from build123d import *

# Parameters (mm, degrees)
ESQUISSE3_R                         = 14.8
BOSS_EXTRU_1_DEPTH                  = 2
BOSS_EXTRU_2_REACH                  = 31.138
R_P_TITION_CIRCULAIRE1_COUNT        = 3
ENL_V_MAT_EXTRU_1_DEPTH             = 30.137604569
ENL_V_MAT_EXTRU_1_DEPTH_BACK        = 30.137604569
ESQUISSE5_R                         = 1.625
PER_AGEAVANC_1_START                = -3.4
PER_AGEAVANC_1_OUTLINE_R            = 3
PER_AGEAVANC_1_OUTLINE_R_2          = 1.625
PER_AGEAVANC_1_DEPTH                = 3.4000121
ENL_V_MAT_EXTRU_2_DEPTH             = 1
ENL_V_MAT_EXTRU_2_DRAFT             = -43
R_P_TITION_CIRCULAIRE2_COPY_1_DEPTH = 1
R_P_TITION_CIRCULAIRE2_COPY_1_DRAFT = -43
R_P_TITION_CIRCULAIRE2_COPY_2_DEPTH = 1
R_P_TITION_CIRCULAIRE2_COPY_2_DRAFT = -43
R_P_TITION_CIRCULAIRE2_COPY_3_DEPTH = 1
R_P_TITION_CIRCULAIRE2_COPY_3_DRAFT = -43


with BuildPart() as part:
    # Esquisse2 → Révolution1 (revolve)
    with BuildSketch(Plane(origin=(0, 0, 0), x_dir=(0, 0, -1), z_dir=(1, 0, 0)), mode=Mode.PRIVATE) as r_volution1_sk:
        Polygon((0, 0), (0, 20), (5, 15), (5, 0), align=None)
    revolve(r_volution1_sk.sketch.rotate(Axis((0, 0, 0), (0, 0, -1)), 90), axis=Axis((0, 0, 0), (0, 0, -1)))

    # Esquisse3 → Boss.-Extru.1 (add)
    with BuildSketch(Plane(origin=(0, 0, -5), x_dir=(-1, 0, 0), z_dir=(0, 0, -1))):
        Circle(ESQUISSE3_R)
    extrude(amount=BOSS_EXTRU_1_DEPTH)

    # Boss.-Extru.2: up to this face of the body (flat: up to its plane)
    boss_extru_2_end = Plane(part.part.faces().sort_by_distance((0, 0, -7))[0])
    # Esquisse4 → Boss.-Extru.2 (add, up to the picked face)
    with BuildSketch(Plane.XY, mode=Mode.PRIVATE) as boss_extru_2_sk1:
        with BuildLine():
            Line((1.5, 19.943670675), (-1.5, 19.943670675))
            Line((-1.5, 19.943670675), (-3.52737474, 14.373504355))
            ThreePointArc((-3.52737474, 14.373504355), (0, 14.8), (3.52737474, 14.373504355))
            Line((3.52737474, 14.373504355), (1.5, 19.943670675))
        make_face()
    boss_extru_2_tool1 = split(extrude(boss_extru_2_sk1.sketch, amount=-BOSS_EXTRU_2_REACH, mode=Mode.PRIVATE), bisect_by=boss_extru_2_end, keep=Keep.BOTH, mode=Mode.PRIVATE)
    boss_extru_2 = boss_extru_2_tool1.solids().sort_by(Axis((0, 16.957577, 0), (0, 0, -1)))[0]
    add(boss_extru_2)

    # Répétition circulaire1: Boss.-Extru.2 ×3 about axis
    r_p_tition_circulaire1_axis = Axis((0, 0, 0), (0, 0, 1))
    for i in range(1, R_P_TITION_CIRCULAIRE1_COUNT):
        add(boss_extru_2.rotate(r_p_tition_circulaire1_axis, i * 360 / R_P_TITION_CIRCULAIRE1_COUNT))

    # Esquisse5 → Enlèv. mat.-Extru.1 (cut, two sides: drawn at the far end of the back side and taken through both)
    with BuildSketch(Plane.XY.offset(-ENL_V_MAT_EXTRU_1_DEPTH_BACK)):
        with Locations((0, 7)):
            Circle(ESQUISSE5_R)
        Circle(ESQUISSE5_R)
        with Locations((7, 0)):
            Circle(ESQUISSE5_R)
        with Locations((0, -7)):
            Circle(ESQUISSE5_R)
        with Locations((-7, 0)):
            Circle(ESQUISSE5_R)
    extrude(amount=ENL_V_MAT_EXTRU_1_DEPTH + ENL_V_MAT_EXTRU_1_DEPTH_BACK, mode=Mode.SUBTRACT)

    # PerçageAvancé1: read off the stored shape, not the designer's step
    # PerçageAvancé1 outline → PerçageAvancé1 (cut)
    # profile 1 of 5: a face of its own
    with BuildSketch(Plane.XY.offset(PER_AGEAVANC_1_START)):
        with Locations((0, -7)):
            Circle(PER_AGEAVANC_1_OUTLINE_R)
        with Locations((0, -7)):
            Circle(PER_AGEAVANC_1_OUTLINE_R_2, mode=Mode.SUBTRACT)
    # profile 2 of 5: a face of its own
    with BuildSketch(Plane.XY.offset(PER_AGEAVANC_1_START)):
        with Locations((7, 0)):
            Circle(PER_AGEAVANC_1_OUTLINE_R)
        with Locations((7, 0)):
            Circle(PER_AGEAVANC_1_OUTLINE_R_2, mode=Mode.SUBTRACT)
    # profile 3 of 5: a face of its own
    with BuildSketch(Plane.XY.offset(PER_AGEAVANC_1_START)):
        Circle(PER_AGEAVANC_1_OUTLINE_R)
        Circle(PER_AGEAVANC_1_OUTLINE_R_2, mode=Mode.SUBTRACT)
    # profile 4 of 5: a face of its own
    with BuildSketch(Plane.XY.offset(PER_AGEAVANC_1_START)):
        with Locations((0, 7)):
            Circle(PER_AGEAVANC_1_OUTLINE_R)
        with Locations((0, 7)):
            Circle(PER_AGEAVANC_1_OUTLINE_R_2, mode=Mode.SUBTRACT)
    # profile 5 of 5: a face of its own
    with BuildSketch(Plane.XY.offset(PER_AGEAVANC_1_START)):
        with Locations((-7, 0)):
            Circle(PER_AGEAVANC_1_OUTLINE_R)
        with Locations((-7, 0)):
            Circle(PER_AGEAVANC_1_OUTLINE_R_2, mode=Mode.SUBTRACT)
    extrude(amount=PER_AGEAVANC_1_DEPTH, mode=Mode.SUBTRACT)


with BuildPart() as enl_v_mat_extru_2_tool:
    # Esquisse9 → Enlèv. mat.-Extru.2 (with draft: the straight prism first)
    with BuildSketch(Plane.XY):
        Polygon((-13.788582233, 11.66726189), (-10.253048327, 4.596194078), (-6.717514421, 4.596194078), (-4.596194078, 6.717514421), (-4.596194078, 10.253048327), (-11.66726189, 13.788582233), align=None)
    extrude(amount=-ENL_V_MAT_EXTRU_2_DEPTH)
    # Enlèv. mat.-Extru.2: the draft: its side faces are tilted about the plane it starts from
    enl_v_mat_extru_2_sides = [enl_v_mat_extru_2_tool.faces().sort_by_distance(p)[0] for p in [
        (-12.02081528, 8.131727984, -0.5),
        (-8.485281374, 4.596194078, -0.5),
        (-5.656854249, 5.656854249, -0.5),
        (-4.596194078, 8.485281374, -0.5),
        (-8.131727984, 12.02081528, -0.5),
        (-12.727922061, 12.727922061, -0.5),
    ]]
    draft(enl_v_mat_extru_2_sides, Plane.XY, ENL_V_MAT_EXTRU_2_DRAFT)


with BuildPart() as part_1:
    add(part.part)

    # Enlèv. mat.-Extru.2: cut by enl_v_mat_extru_2_tool
    add(enl_v_mat_extru_2_tool.part, mode=Mode.SUBTRACT)


with BuildPart() as r_p_tition_circulaire2_copy_1_tool:
    # Répétition circulaire2 copy 1 sketch → Répétition circulaire2 copy 1 (with draft: the straight prism first)
    with BuildSketch(Plane(origin=(0, 0, 0), x_dir=(0, 1, 0), z_dir=(0, 0, 1))):
        Polygon((-13.788582233, 11.66726189), (-10.253048327, 4.596194078), (-6.717514421, 4.596194078), (-4.596194078, 6.717514421), (-4.596194078, 10.253048327), (-11.66726189, 13.788582233), align=None)
    extrude(amount=-R_P_TITION_CIRCULAIRE2_COPY_1_DEPTH)
    # Répétition circulaire2 copy 1: the draft: its side faces are tilted about the plane it starts from
    r_p_tition_circulaire2_copy_1_sides = [r_p_tition_circulaire2_copy_1_tool.faces().sort_by_distance(p)[0] for p in [
        (-8.131727984, -12.02081528, -0.5),
        (-4.596194078, -8.485281374, -0.5),
        (-5.656854249, -5.656854249, -0.5),
        (-8.485281374, -4.596194078, -0.5),
        (-12.02081528, -8.131727984, -0.5),
        (-12.727922061, -12.727922061, -0.5),
    ]]
    draft(r_p_tition_circulaire2_copy_1_sides, Plane(origin=(0, 0, 0), x_dir=(0, 1, 0), z_dir=(0, 0, 1)), R_P_TITION_CIRCULAIRE2_COPY_1_DRAFT)


with BuildPart() as part_2:
    add(part_1.part)

    # Répétition circulaire2 copy 1: cut by r_p_tition_circulaire2_copy_1_tool
    add(r_p_tition_circulaire2_copy_1_tool.part, mode=Mode.SUBTRACT)


with BuildPart() as r_p_tition_circulaire2_copy_2_tool:
    # Répétition circulaire2 copy 2 sketch → Répétition circulaire2 copy 2 (with draft: the straight prism first)
    with BuildSketch(Plane(origin=(0, 0, 0), x_dir=(-1, 0, 0), z_dir=(0, 0, 1))):
        Polygon((-13.788582233, 11.66726189), (-10.253048327, 4.596194078), (-6.717514421, 4.596194078), (-4.596194078, 6.717514421), (-4.596194078, 10.253048327), (-11.66726189, 13.788582233), align=None)
    extrude(amount=-R_P_TITION_CIRCULAIRE2_COPY_2_DEPTH)
    # Répétition circulaire2 copy 2: the draft: its side faces are tilted about the plane it starts from
    r_p_tition_circulaire2_copy_2_sides = [r_p_tition_circulaire2_copy_2_tool.faces().sort_by_distance(p)[0] for p in [
        (12.02081528, -8.131727984, -0.5),
        (8.485281374, -4.596194078, -0.5),
        (5.656854249, -5.656854249, -0.5),
        (4.596194078, -8.485281374, -0.5),
        (8.131727984, -12.02081528, -0.5),
        (12.727922061, -12.727922061, -0.5),
    ]]
    draft(r_p_tition_circulaire2_copy_2_sides, Plane(origin=(0, 0, 0), x_dir=(-1, 0, 0), z_dir=(0, 0, 1)), R_P_TITION_CIRCULAIRE2_COPY_2_DRAFT)


with BuildPart() as part_3:
    add(part_2.part)

    # Répétition circulaire2 copy 2: cut by r_p_tition_circulaire2_copy_2_tool
    add(r_p_tition_circulaire2_copy_2_tool.part, mode=Mode.SUBTRACT)


with BuildPart() as r_p_tition_circulaire2_copy_3_tool:
    # Répétition circulaire2 copy 3 sketch → Répétition circulaire2 copy 3 (with draft: the straight prism first)
    with BuildSketch(Plane(origin=(0, 0, 0), x_dir=(0, -1, 0), z_dir=(0, 0, 1))):
        Polygon((-13.788582233, 11.66726189), (-10.253048327, 4.596194078), (-6.717514421, 4.596194078), (-4.596194078, 6.717514421), (-4.596194078, 10.253048327), (-11.66726189, 13.788582233), align=None)
    extrude(amount=-R_P_TITION_CIRCULAIRE2_COPY_3_DEPTH)
    # Répétition circulaire2 copy 3: the draft: its side faces are tilted about the plane it starts from
    r_p_tition_circulaire2_copy_3_sides = [r_p_tition_circulaire2_copy_3_tool.faces().sort_by_distance(p)[0] for p in [
        (8.131727984, 12.02081528, -0.5),
        (4.596194078, 8.485281374, -0.5),
        (5.656854249, 5.656854249, -0.5),
        (8.485281374, 4.596194078, -0.5),
        (12.02081528, 8.131727984, -0.5),
        (12.727922061, 12.727922061, -0.5),
    ]]
    draft(r_p_tition_circulaire2_copy_3_sides, Plane(origin=(0, 0, 0), x_dir=(0, -1, 0), z_dir=(0, 0, 1)), R_P_TITION_CIRCULAIRE2_COPY_3_DRAFT)


with BuildPart() as part_4:
    add(part_3.part)

    # Répétition circulaire2 copy 3: cut by r_p_tition_circulaire2_copy_3_tool
    add(r_p_tition_circulaire2_copy_3_tool.part, mode=Mode.SUBTRACT)


solid = part_4.part
Read the model definition and answer for the solid it produces. Units are mm, in the model's axes. A direction names the side the tool comes from. Coordinates: 2 decimals unless noted, no trailing zeros. Loops run counter-clockwise (first coordinate to the right, second up) from the corner with the lowest first, then second, coordinate; pieces in that order, holes last. Notation, with made-up numbers: (-33, 81) - (-9, 81) arc R23 ccw to (-9, 112) - close; hole circle Ø3 at (30, 77.5). An arc over 180 degrees is marked (long way). Answer in a Markdown table with one row per item.
Q1. Given P1, Ø3.5, axis at x = 0.5, z = -2, coming from the +Y side; P2, Ø3.5, axis at x = 9.5, y = 8.5, coming from the +Z side; P3, Ø1.8, axis at x = -8, y = -0.5, coming from the +Z side, each flat-ended and moving along its own axis, determine where each tip first touches the part or whether it passes through.
Here are the results:
| item | result |
|---|---|
| P1 | stops at y = 19.94 |
| P2 | stops at z = -0.72 |
| P3 | stops at z = -3.4 |
Q2. The mould has two halves that part along X. Classify faces 1 (the flat face through (-4, 4, 0)), 2 (the cylindrical face through (-12.9, 7.255, -5.986)), 3 (the flat face through (-5.056, -8.51, -0.493)): pulls with the +X half, pulls with the -X half, needs draft (parallel to the pull), parting line crosses it, or undercut.
Here are the results:
| item | result |
|---|---|
| face 1 | needs draft |
| face 2 | pulls with the -X half |
| face 3 | undercut |
Q3. Straight lines are drawn through the part: line 1 along X through (y, z) = (0, -6.15) (3 decimals); line 2 along Y through (x, z) = (0, -1.9); line 3 along Y through (x, z) = (0, -1.25). For each, find the intervals that lie inside material, in ascending order. Write a range as [from, to].
Here are the results:
| item | result |
|---|---|
| line 1 | x = [-14.8, -8.625], [-5.375, -1.625], [1.625, 5.375], [8.625, 14.8] |
| line 2 | y = [-18.1, -10], [-4, -3], [3, 4], [10, 19.94] |
| line 3 | y = [-18.75, -10], [-4, -3], [3, 4], [10, 19.94] |
Q4. For faces 4 (the cylindrical face through (0.2, -14.8, -6)), 5 (the flat face through (1.3, -8.3, -3.4)), 6 (the cylindrical face through (-0.21, -5.39, -5.23)), determine the directions among +Z, -Z, +X, -X, +Y, -Y from which every point of the face is accessible in a straight line to the end or side of a thin tool.
Here are the results:
| item | result |
|---|---|
| face 4 | -Z, -Y |
| face 5 | +Z |
| face 6 | +Z, -Z |
Q5. Find section D-D on z = -2. Write down the section's boundary in (x, y), plus the area to 3 significant figures.
Here are the results:
| item | result |
|---|---|
| outline | (-18.02, -8.67) - (-16.52, -11.27) - (-14.34, -10.89) arc R18 ccw to (14.34, -10.89) - (16.52, -11.27) - (18.02, -8.67) - (16.59, -6.97) arc R18 ccw to (2.26, 17.86) - (1.5, 19.94) - (-1.5, 19.94) - (-2.26, 17.86) arc R18 ccw to (-16.59, -6.97) - close; hole circle Ø6 at (-7, 0); hole circle Ø6 at (0, -7); hole circle Ø6 at (0, 0); hole circle Ø6 at (0, 7); hole circle Ø6 at (7, 0) |
| area | 899 mm^2 |
Q6. Find section A-A on x = 0. Count the separate pieces of the cut face and the enclosed holes in it, plus the area to 3 significant figures.
Here are the results:
| item | result |
|---|---|
| separate pieces | 4 |
| enclosed holes | 0 |
| area | 160 mm^2 |
